Geometry: see drawing. Coordinates: mm, zero at the bounding-box minimum. A direction names the side the tool comes from. Coordinates: 2 decimals unless noted, no trailing zeros. Write each loop counter-clockwise with the first axis right and the second up, starting at its lowest first coordinate (ties: lowest second). Pieces come first, ordered by that corner, then holes.
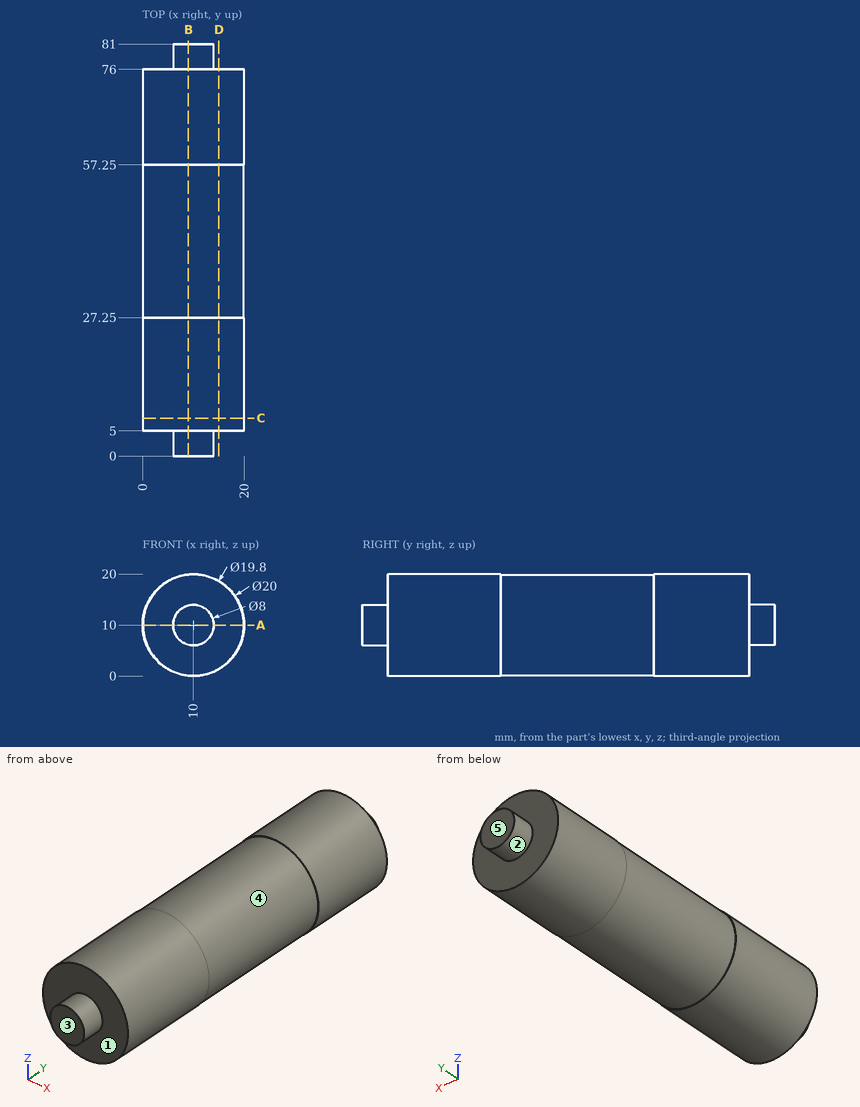
Item 1: Section A-A, the plane z = 10. Output: boundary loops of the cut face in (x, y).
Derived:
outline: (0, 5) - (6, 5) - (6, 0) - (14, 0) - (14, 5) - (20, 5) - (20, 27.25) - (19.9, 27.25) - (19.9, 57.25) - (20, 57.25) - (20, 76) - (14, 76) - (14, 81) - (6, 81) - (6, 76) - (0, 76) - (0, 57.25) - (0.1, 57.25) - (0.1, 27.25) - (0, 27.25) - close
Item 2: Set-up query: the marked faces 1, 2, 3, 4 and 5. Return all of +Z, -Z, +X, -X, +Y, -Y with unobstructed straight access to the full face (end or side cutting, diameter ignored); none if empty.
Derived:
face 1: -Y
face 2: +Y
face 3: +Z, -Z, +X, -X, -Y
face 4: none
face 5: +Z, -Z, +X, -X, +Y
Item 3: Section C-C, the plane y = 7.5. Output: boundary loops of the cut face in (x, z).
Derived:
outline: circle Ø20 at (10, 10)
Item 4: Material intervals for probe 1 along Y at (x, z) = (14, 17); probe 2 along X at (y, z) = (65, 7.5); probe 3 along X at (y, z) = (75.5, 1.25), sorted ascending.
Derived:
probe 1: y = 5 to 76
probe 2: x = 0.32 to 19.68
probe 3: x = 5.16 to 14.84
Item 5: Section D-D, the plane x = 15. Output: boundary loops of the cut face in (y, z), plus the area to 3 significant figures.
Derived:
outline: (5, 1.34) - (27.25, 1.34) - (27.25, 1.46) - (57.25, 1.46) - (57.25, 1.34) - (76, 1.34) - (76, 18.66) - (57.25, 18.66) - (57.25, 18.54) - (27.25, 18.54) - (27.25, 18.66) - (5, 18.66) - close
area: 1,220 mm2
Item 6: Pin query (flat end, axial travel): pin 1 (4 mm diameter, centred on y = 8, z = 14, fed in from -X); pin 2 (6 mm diameter, centred on x = 3, y = 58, fed in from -Z); pin 3 (1 mm diameter, centred on y = 28.5, z = 15.5, fed in from +X). Return the tip coordinate at first contact, or that it passes through.
Derived:
pin 1: stops at x = 0.2
pin 2: stops at z = 0.83
pin 3: stops at x = 18.54
Item 7: Section B-B, the plane x = 9. Output: boundary loops of the cut face in (y, z), plus the area to 3 significant figures.
Derived:
outline: (0, 6.13) - (5, 6.13) - (5, 0.05) - (27.25, 0.05) - (27.25, 0.15) - (57.25, 0.15) - (57.25, 0.05) - (76, 0.05) - (76, 6.13) - (81, 6.13) - (81, 13.87) - (76, 13.87) - (76, 19.95) - (57.25, 19.95) - (57.25, 19.85) - (27.25, 19.85) - (27.25, 19.95) - (5, 19.95) - (5, 13.87) - (0, 13.87) - close
area: 1,480 mm2
